```python
from build123d import *

# Parameters (mm, degrees)
EXTRUDE_1_DEPTH     = 5
FILLET_1_R          = 20
EXTRUDE_START       = 3
EXTRUDE_2_DEPTH     = 3
SKETCH_5_W          = 424.898907654
SKETCH_5_H          = 342.867142677
CUT_EXTRUDE_2_DEPTH = 13


with BuildPart() as part:
    # 草圖1 → 填料-伸長1 (new body)
    with BuildSketch(Plane(origin=(0, 0, 0), x_dir=(1, 0, 0), z_dir=(0, 1, 0))):
        Polygon((-90.122176988, 0), (90.122176988, 0), (165.122176988, 129.903810568), (75, 286), (-75, 286), (-165.122176988, 129.903810568), align=None)
    extrude(amount=EXTRUDE_1_DEPTH)

    # 圓角1
    fillet_1_edges = [part.edges().sort_by_distance(p)[0] for p in [
        (-165.122176988, 2.5, -129.903810568),
        (-75, 2.5, -286),
        (75, 2.5, -286),
        (165.122176988, 2.5, -129.903810568),
        (90.122176988, 2.5, 0),
        (-90.122176988, 2.5, 0),
    ]]
    fillet(fillet_1_edges, radius=FILLET_1_R)

    # 草圖3 → 填料-伸長2 (add)
    with BuildSketch(Plane(origin=(0, 5, 0), x_dir=(1, 0, 0), z_dir=(0, 1, 0)).offset(EXTRUDE_START)):
        with BuildLine():
            Line((-159.348674296, 119.903810568), (-140.378315376, 87.04618508))
            ThreePointArc((-140.378315376, 87.04618508), (-129.903810568, 64.903810568), (-115.965204144, 44.761436056))
            Line((-115.965204144, 44.761436056), (-95.89567968, 10))
            ThreePointArc((-95.89567968, 10), (-88.575171604, 2.679491924), (-78.575171604, 0))
            Line((-78.575171604, 0), (-54.101051641, 0))
            ThreePointArc((-54.101051641, 0), (0, -10.096189432), (54.101051641, 0))
            Line((54.101051641, 0), (78.575171604, 0))
            ThreePointArc((78.575171604, 0), (88.575171604, 2.679491924), (95.89567968, 10))
            Line((95.89567968, 10), (115.965204144, 44.761436056))
            ThreePointArc((115.965204144, 44.761436056), (129.903810568, 64.903810568), (140.378315376, 87.04618508))
            Line((140.378315376, 87.04618508), (159.348674296, 119.903810568))
            ThreePointArc((159.348674296, 119.903810568), (162.028166221, 129.903810568), (159.348674296, 139.903810568))
            Line((159.348674296, 139.903810568), (148.905382636, 157.992122322))
            ThreePointArc((148.905382636, 157.992122322), (129.903810568, 214.903810568), (90.117628809, 259.815498813))
            Line((90.117628809, 259.815498813), (80.773502692, 276))
            ThreePointArc((80.773502692, 276), (73.452994616, 283.320508076), (63.452994616, 286))
            Line((63.452994616, 286), (33.998579873, 286))
            ThreePointArc((33.998579873, 286), (0, 289.903810568), (-33.998579873, 286))
            Line((-33.998579873, 286), (-63.452994616, 286))
            ThreePointArc((-63.452994616, 286), (-73.452994616, 283.320508076), (-80.773502692, 276))
            Line((-80.773502692, 276), (-90.117628809, 259.815498813))
            ThreePointArc((-90.117628809, 259.815498813), (-129.903810568, 214.903810568), (-148.905382636, 157.992122322))
            Line((-148.905382636, 157.992122322), (-159.348674296, 139.903810568))
            ThreePointArc((-159.348674296, 139.903810568), (-162.028166221, 129.903810568), (-159.348674296, 119.903810568))
        make_face()
    extrude(amount=-EXTRUDE_2_DEPTH)

    # 草圖5 → 除料-伸長2 (cut)
    with BuildSketch(Plane.XZ.offset(-5)):
        with Locations((0.961309746, -138.62206424)):
            Rectangle(SKETCH_5_W, SKETCH_5_H)
    extrude(amount=CUT_EXTRUDE_2_DEPTH, mode=Mode.SUBTRACT)


solid = part.part
```
Geometry check sheet. Reference: the model listing, model coordinates, mm. Coordinates: 2 decimals unless noted, no trailing zeros. Order: outer loops, then holes, each group sorted by start corner. A loop starts at its lowest first (then second) coordinate and runs counter-clockwise, first axis right, second up. Notation, with made-up numbers: M 27.25,-39.5 L 42.25,-39.5 A18 ccw 42.25,-10.5 Z; hole C -0.5,-27 d9. An arc over 180 degrees is marked long. One line per question, with ' | ' between items. Start each with the question number.
Item 1: Gauge pin test, flat ends, axial feed: pin 1 (0.9 mm diameter, centred on x = -71.5, y = 6.5, fed in from +Z); pin 2 (1.5 mm diameter, centred on y = 6, z = -121, fed in from +X); pin 3 (0.9 mm diameter, centred on x = -49.5, y = 7, fed in from -Z). Record the tip position at first contact, or that the pin passes through.
Item 2: Cross-section at C-C on x = -135. Enter the section's corners in (y, z).
Item 3: Material ranges on L1, parallel to Z at x = 62, y = 6.4; L2, parallel to X at y = 7.35, z = -207; L3, parallel to X at y = 6.55, z = -215, recorded low to high. Write a range as [from, to].
Item 4: Cross-section at A-A on y = 6.75. Enter the section's corners in (x, z).
Item 5: Cross-section at B-B on z = -244.5. Enter the section's corners in (x, y).
Findings:
1) pin 1: stops at z = 0 | pin 2: stops at x = 160.29 | pin 3: stops at z = -286
2) outline: M 5,-205.29 L 8,-205.29 L 8,-74.52 L 5,-74.52 Z
3) L1: z = [-286, 0] | L2: x = [-134.16, 134.16] | L3: x = [-129.85, 129.85]
4) outline: M -159.35,-139.9 L -148.91,-157.99 A150 ccw -90.12,-259.82 L -80.77,-276 A20 ccw -63.45,-286 L -34,-286 A150 ccw 34,-286 L 63.45,-286 A20 ccw 80.77,-276 L 90.12,-259.82 A150 ccw 148.91,-157.99 L 159.35,-139.9 A20 ccw 159.35,-119.9 L 140.38,-87.05 A150 ccw 115.97,-44.76 L 95.9,-10 A20 ccw 78.58,0 L 54.1,0 A150 ccw -54.1,0 L -78.58,0 A20 ccw -95.9,-10 L -115.97,-44.76 A150 ccw -140.38,-87.05 L -159.35,-119.9 A20 ccw Z
5) outline: M -107.52,5 L 107.52,5 L 107.52,8 L -107.52,8 Z
